The listing builds one solid part. Answer for the finished solid, in the listing's coordinates (mm). A direction names the side the tool comes from. Give positions to 0.01 mm unless a question says otherwise; leave off trailing zeros. Loops run counter-clockwise (first coordinate to the right, second up) from the corner with the lowest first, then second, coordinate; pieces in that order, holes last. Notation, with made-up numbers: (54, 5.25) - (94, 5.25) arc R18 ccw to (94, 34.25) - close; hole circle Ø2 at (5, 37.25). An arc over 180 degrees is marked (long way). Answer in a Markdown table with one row per item. Add a question column.
Autodesk Inventor part; units mm, degrees
ref_plane "YZ Plane" through (0, 0, 0) normal (1, 0, 0) x (0, 1, 0)
ref_plane "XZ Plane" through (0, 0, 0) normal (0, 1, 0) x (-1, 0, 0)
ref_plane "XY Plane" through (0, 0, 0) normal (0, 0, 1) x (1, 0, 0)
sketch "Sketch1" plane through (0, 0, 0) normal (0, 0, 1) x (1, 0, 0)
  line L0 (-257.8464, 52.4999) -> (-100.2151, 52.4999) construction
  line L1 (-100.2151, 52.4999) -> (-100.2151, -56.2898) construction
  line L2 (-100.2151, -56.2898) -> (-257.8464, -56.2898) construction
  line L3 (-257.8464, -56.2898) -> (-257.8464, 52.4999) construction
  line L4 (40, -20) -> (40, 20)
  line L5 (-40, 20) -> (-40, -20)
  line L6 (-6.1649, 0) -> (6.1649, 0)
  line L7 (-30, 20) -> (-6.1649, 0)
  line L8 (30, 20) -> (6.1649, 0)
  line L9 (40, 20) -> (30, 20)
  line L10 (-30, 20) -> (-40, 20)
  arc A0 (-26.087, -54.3676) -> (26.087, -54.3676) centre (0, -81.3068) ccw
  arc A1 (-26.087, -54.3676) -> (-40, -20) centre (-40, -40) ccw
  arc A2 (40, -20) -> (26.087, -54.3676) centre (40, -40) ccw
  point P0 (0, 0)
  point P1 (-24.7924, -52.9895)
  point P2 (24.7924, -52.9895)
  dimension "d7" = 80
  dimension "d8" = 40
  dimension "d9" = 10
  dimension "d10" = 10
  dimension "d16" = 75
  dimension "d17" = 20
extrude "Extrusion1" add sketch "Sketch1" along normal blind 50
sketch "Sketch2" plane through (0, 0, 50) normal (0, 0, 1) x (1, 0, 0)
  arc A0 (-26.087, -54.3676) -> (26.087, -54.3676) centre (0, -81.3068) ccw
  circle A1 centre (0, -81.3068) radius 22.5
  point P0 (0, 0)
  dimension "d23" = 45
extrude "Extrusion2" cut sketch "Sketch2" against normal through all
sketch "Sketch3" plane through (-6.1649, 0, 0) normal (0, 1, 0) x (1, 0, 0)
  line L0 (12.3299, -50) -> (0, -50)
  line L1 (0, 0) -> (0, -50)
  line L2 (12.3299, 0) -> (12.3299, -50)
  circle A0 centre (6.1649, -25) radius 6.165
  point P0 (6.1649, 0)
  point P1 (12.3299, -24.9702)
  point P2 (0, -24.9702)
  point P3 (0, -25.0298)
  point P4 (12.3299, -25.0298)
  dimension "d26" = 12.3299
  dimension "d27" = 12.33
extrude "Extrusion3" cut sketch "Sketch3" against normal blind 60 contours A0
properties part number "cad@39"
(1) A cutting plane is placed at C-C on x = -27.5. Determine the outline of the cut face in (y, z).
(2) The mould has two halves that part along X. Classify faces 4 (the face through (21.34, -32.8, 24.65)), 5 (the face through (-18.2, 10.1, 24.6)), 6 (the face through (1.245, -118.786, 24.65)): pulls with the +X half, pulls with the -X half, needs draft (parallel to the pull), parting line crosses it, or undercut.
(3) Given pin 1 Ø2 at (x, z) = (-29.5, 41) entering from -Y; pin 2 Ø10 at (x, z) = (-24.5, 11) entering from -Y; pin 3 Ø5 at (y, z) = (-30.5, 21.5) entering from -X, each flat-ended and moving along its own axis, determine where each tip first touches the part or whether it passes through.
(4) A cutting plane is placed at B-B on y = -64. Determine the outline of the cut face in (x, z), plus the area to 3 significant figures.
(5) A cutting plane is placed at D-D on z = 5.5. Determine the outline of the cut face in (x, y).
(6) A cutting plane is placed at A-A on x = 0. Determine the outline of the cut face in (y, z) (3 decimals).
(7) Find the intervals of material crossed by line 1 along Y through (x, z) = (1, 39); line 2 along Z through (x, y) = (0, -39.5) (3 decimals); line 3 along X through (y, z) = (-83.5, 15), in increasing order. Write a range as [from, to].
(8) A tool of negligible diameter and unlimited length cuts with its end or side. For faces 1 (the face through (-1, -48, 0)), 2 (the face through (0, 0, 10)), 3 (the face through (-0.803, -29.417, 18.887)), from which of +Z, -Z, +X, -X, +Y, -Y can it reach the whole face along a straight path? Write none if from no direction.
Evaluation:
| question | item | result |
|---|---|---|
| 1 | outline | (-106.8, 0) - (-55.81, 0) - (-55.81, 50) - (-106.8, 50) - close; (-24.39, 0) - (17.9, 0) - (17.9, 50) - (-24.39, 50) - close |
| 2 | face 4 | pulls with the +X half |
| 2 | face 5 | undercut |
| 2 | face 6 | parting line crosses it |
| 3 | pin 1 | stops at y = -105.68 |
| 3 | pin 2 | stops at y = -113.34 |
| 3 | pin 3 | stops at x = -24 |
| 4 | outline | (-33.27, 0) - (-14.38, 0) - (-14.38, 50) - (-33.27, 50) - close; (14.38, 0) - (33.27, 0) - (33.27, 50) - (14.38, 50) - close |
| 4 | area | 1,890 mm² |
| 5 | outline | (-40, -20) arc R20 cw to (-26.09, -54.37) arc R37.5 ccw (long way) to (26.09, -54.37) arc R20 cw to (40, -20) - (40, 20) - (30, 20) - (6.16, 0) - (-6.16, 0) - (-30, 20) - (-40, 20) - close; hole circle Ø45 at (0, -81.31) |
| 6 | outline | (-118.807, 0) - (-103.807, 0) - (-103.807, 50) - (-118.807, 50) - close; (-58.807, 0) - (0, 0) - (0, 18.835) - (-58.807, 18.835) - close; (-58.807, 31.165) - (0, 31.165) - (0, 50) - (-58.807, 50) - close |
| 7 | line 1 | y = [-118.79, -103.78], [-58.83, 0] |
| 7 | line 2 | z = [0, 18.835], [31.165, 50] |
| 7 | line 3 | x = [-37.44, -22.39], [22.39, 37.44] |
| 8 | face 1 | -Z, +X, -X, +Y, -Y |
| 8 | face 2 | +Z, -Z, +Y |
| 8 | face 3 | +Y |
